Check sheet for the modelled part. Datum: model origin and axes. Units: mm. A direction names the side the tool comes from. Round coordinates to 2 decimals unless told otherwise and drop trailing zeros. Loops run counter-clockwise (first coordinate to the right, second up) from the corner with the lowest first, then second, coordinate; pieces in that order, holes last. Notation, with made-up numbers: (-35, 15.5) -> (-24, 15.5) arc R23 ccw to (-24, 46.5) -> close; hole circle Ø11 at (80.5, -24). An arc over 180 degrees is marked (long way). Use one line per item in the form item = value. Start each with the question number.
(1) Sectioned sample at C-C (z = 36.5). Record the cut outline in (x, y), and give its area (3 significant figures).
(2) Sectioned sample at A-A (z = 22). Record the cut outline in (x, y).
(3) Material ranges on probe 1 along Y at (x, z) = (-21.5, 2.15); probe 2 along X at (y, z) = (13, 8.5); probe 3 along Z at (x, y) = (-24, 0.5), recorded low to high. Write a range as [from, to].
(4) Set-up check for faces 5 (the flat face through (0, 0, 0)), 6 (the cylindrical face through (0.253, -11.497, 26.381)), 7 (the cylindrical face through (22.9, 23.69, 2.46)), 8 (the flat face through (-8.5, 8, 16)), 9 (the flat face through (16.5, 8, 23)): record each of +Z, -Z, +X, -X, +Y, -Y from which the full face is reachable in a straight line by a thin tool's end or side.
(5) Draft check along X on faces 1 (the cylindrical face through (-0.363, -16.496, 22.748)), 2 (the flat face through (13, 16.5, 23)), 3 (the flat face through (0, 0, 5)), 4 (the flat face through (11.5, 8, 8)). Enter one of: released by +X, released by -X, zero draft, split by the parting line, or undercut.
(6) Go/stop test with flat-tipped pins: pin 1 (7 mm diameter, centred on x = 3.5, y = 5.5, fed in from +Z); pin 2 (12 mm diameter, centred on x = 12, z = 23.5, fed in from +Y); pin 3 (3.5 mm diameter, centred on y = 8.5, z = 40, fed in from -X). Record where each tip stops, or that it passes through.
from build123d import *

# Parameters (mm, degrees)
F0_R     = 2.6
F1_DEPTH = 5
F3_DEPTH = 36
F6_DEPTH = 3
F9_DEPTH = 3
F10_SIZE = 2.99999


# Not quite as in the source:
# - a fillet or chamfer is up to 0.001 mm smaller than in the source, because OpenCascade refuses the exact size


with BuildPart() as f1:
    # F0 (on Top) → F1 (new body)
    with BuildSketch(Plane.XY):
        with BuildLine():
            Line((21.5, 26.5), (-21.5, 26.5))
            ThreePointArc((-21.5, 26.5), (-17.9644660941, 25.0355339059), (-16.5, 21.5))
            ThreePointArc((-16.5, 21.5), (-21.5, 16.5), (-26.5, 21.5))
            Line((-26.5, 21.5), (-26.5, -21.5))
            ThreePointArc((-26.5, -21.5), (-21.5, -16.5), (-16.5, -21.5))
            ThreePointArc((-16.5, -21.5), (-17.9644660941, -25.0355339059), (-21.5, -26.5))
            Line((-21.5, -26.5), (21.5, -26.5))
            ThreePointArc((21.5, -26.5), (17.9644660941, -17.9644660941), (26.5, -21.5))
            Line((26.5, -21.5), (26.5, 21.5))
            ThreePointArc((26.5, 21.5), (17.9644660941, 17.9644660941), (21.5, 26.5))
        make_face()
        with BuildLine():
            Line((-11.5, 16.5), (-11.5, 0))
            ThreePointArc((-11.5, 0), (0, -11.5), (11.5, 0))
            Line((11.5, 0), (11.5, 16.5))
            Line((11.5, 16.5), (16.5, 16.5))
            Line((16.5, 16.5), (16.5, 0))
            ThreePointArc((16.5, 0), (0, -16.5), (-16.5, 0))
            Line((-16.5, 0), (-16.5, 16.5))
            Line((-16.5, 16.5), (-11.5, 16.5))
        make_face(mode=Mode.SUBTRACT)
        with BuildLine():
            ThreePointArc((11.5, 0), (0, -11.5), (-11.5, 0))
            Line((-11.5, 0), (-11.5, 16.5))
            Line((-11.5, 16.5), (-16.5, 16.5))
            Line((-16.5, 16.5), (-16.5, 0))
            ThreePointArc((-16.5, 0), (0, -16.5), (16.5, 0))
            Line((16.5, 0), (16.5, 16.5))
            Line((16.5, 16.5), (11.5, 16.5))
            Line((11.5, 16.5), (11.5, 0))
        make_face()
        with BuildLine():
            ThreePointArc((-16.5, 21.5), (-17.9644660941, 25.0355339059), (-21.5, 26.5))
            ThreePointArc((-21.5, 26.5), (-25.0355339059, 25.0355339059), (-26.5, 21.5))
            ThreePointArc((-26.5, 21.5), (-21.5, 16.5), (-16.5, 21.5))
        make_face()
        with Locations((-21.5, 21.5)):
            Circle(F0_R, mode=Mode.SUBTRACT)
        with BuildLine():
            ThreePointArc((-16.5, -21.5), (-21.5, -16.5), (-26.5, -21.5))
            ThreePointArc((-26.5, -21.5), (-25.0355339059, -25.0355339059), (-21.5, -26.5))
            ThreePointArc((-21.5, -26.5), (-17.9644660941, -25.0355339059), (-16.5, -21.5))
        make_face()
        with Locations((-21.5, -21.5)):
            Circle(F0_R, mode=Mode.SUBTRACT)
        with BuildLine():
            ThreePointArc((21.5, -26.5), (25.0355339059, -25.0355339059), (26.5, -21.5))
            ThreePointArc((26.5, -21.5), (17.9644660941, -17.9644660941), (21.5, -26.5))
        make_face()
        with Locations((21.5, -21.5)):
            Circle(F0_R, mode=Mode.SUBTRACT)
        with BuildLine():
            ThreePointArc((26.5, 21.5), (25.0355339059, 25.0355339059), (21.5, 26.5))
            ThreePointArc((21.5, 26.5), (17.9644660941, 17.9644660941), (26.5, 21.5))
        make_face()
        with Locations((21.5, 21.5)):
            Circle(F0_R, mode=Mode.SUBTRACT)
    extrude(amount=F1_DEPTH)

    # F2 (on face) → F3 (join)
    with BuildSketch(Plane.XY.offset(5)):
        with BuildLine():
            ThreePointArc((11.5, 0), (0, -11.5), (-11.5, 0))
            Line((-11.5, 0), (-11.5, 16.5))
            Line((-11.5, 16.5), (-16.5, 16.5))
            Line((-16.5, 16.5), (-16.5, 0))
            ThreePointArc((-16.5, 0), (0, -16.5), (16.5, 0))
            Line((16.5, 0), (16.5, 16.5))
            Line((16.5, 16.5), (11.5, 16.5))
            Line((11.5, 16.5), (11.5, 0))
        make_face()
    extrude(amount=F3_DEPTH)

    # F5 (on offset) → F6 (join)
    with BuildSketch(Plane.XY.offset(15)):
        with BuildLine():
            Line((-11.5, 16.5), (-11.5, 0))
            ThreePointArc((-11.5, 0), (0, -11.5), (11.5, 0))
            Line((11.5, 0), (11.5, 16.5))
            Line((11.5, 16.5), (8.5, 16.5))
            Line((8.5, 16.5), (8.5, 0))
            ThreePointArc((8.5, 0), (0, -8.5), (-8.5, 0))
            Line((-8.5, 0), (-8.5, 16.5))
            Line((-8.5, 16.5), (-11.5, 16.5))
        make_face()
    extrude(amount=F6_DEPTH)

    # F8 (on offset) → F9 (join)
    with BuildSketch(Plane.XY.offset(38)):
        with BuildLine():
            Line((-11.5, 16.5), (-11.5, 0))
            ThreePointArc((-11.5, 0), (0, -11.5), (11.5, 0))
            Line((11.5, 0), (11.5, 16.5))
            Line((11.5, 16.5), (8.5, 16.5))
            Line((8.5, 16.5), (8.5, 0))
            ThreePointArc((8.5, 0), (0, -8.5), (-8.5, 0))
            Line((-8.5, 0), (-8.5, 16.5))
            Line((-8.5, 16.5), (-11.5, 16.5))
        make_face()
    extrude(amount=F9_DEPTH)

    # F10 (size 3 in the source; OpenCascade refuses exactly that, so slightly less here)
    f10_edges = [f1.edges().sort_by_distance(p)[0] for p in [
        (-11.5, 8.25, 38),
        (-11.5, 8.25, 15),
    ]]
    chamfer(f10_edges, length=F10_SIZE)


solid = f1.part
Checks:
q1.outline = (-16.5, 0) arc R16.5 ccw to (16.5, 0) -> (16.5, 16.5) -> (10, 16.5) -> (10, 0) arc R10 cw to (-10, 0) -> (-10, 16.5) -> (-16.5, 16.5) -> close
q1.area = 485 mm2
q2.outline = (-16.5, 0) arc R16.5 ccw to (16.5, 0) -> (16.5, 16.5) -> (11.5, 16.5) -> (11.5, 0) arc R11.5 cw to (-11.5, 0) -> (-11.5, 16.5) -> (-16.5, 16.5) -> close
q3.probe_1 = [-26.5, -24.1], [-18.9, 18.9], [24.1, 26.5]
q3.probe_2 = [-16.5, -11.5], [11.5, 16.5]
q3.probe_3 = [0, 5]
q4.face_5 = -Z, +X, -X, +Y, -Y
q4.face_6 = +Y
q4.face_7 = +Z, -Z
q4.face_8 = +Z, +Y
q4.face_9 = +Z, +X, +Y, -Y
q5.face_1 = split by the parting line
q5.face_2 = zero draft
q5.face_3 = undercut
q5.face_4 = undercut
q6.pin_1 = 5
q6.pin_2 = 16.5
q6.pin_3 = -16.5
